from build123d import *

# Parameters (mm, degrees)
F0_R     = 14.25
F1_DEPTH = 83
F2_W     = 44.470418
F2_H     = 54.147916
F3_DEPTH = 12.5
F4_R     = 14.971262
F4_R_2   = 11
F5_DEPTH = 14


with BuildPart() as f1:
    # F0 (on Top) → F1 (new body)
    with BuildSketch(Plane.XY):
        with BuildLine():
            ThreePointArc((-11, 11.61895), (-6.324555, -14.696938), (16, 0))
            ThreePointArc((16, 0), (14.696938, 6.324555), (11, 11.61895))
            ThreePointArc((11, 11.61895), (0, 16), (-11, 11.61895))
        make_face()
        Circle(F0_R, mode=Mode.SUBTRACT)
        with BuildLine():
            ThreePointArc((-11, 76.61895), (0, 65.61895), (11, 76.61895))
            ThreePointArc((11, 76.61895), (10.797649, 78.719137), (10.198039, 80.742056))
            Line((10.198039, 80.742056), (8, 80.742056))
            ThreePointArc((8, 80.742056), (0, 67.61895), (-8, 80.742056))
            Line((-8, 80.742056), (-10.198039, 80.742056))
            ThreePointArc((-10.198039, 80.742056), (-10.797649, 78.719137), (-11, 76.61895))
        make_face()
        with BuildLine():
            ThreePointArc((-11, 11.61895), (0, 16), (11, 11.61895))
            Line((11, 11.61895), (11, 76.61895))
            ThreePointArc((11, 76.61895), (0, 65.61895), (-11, 76.61895))
            Line((-11, 76.61895), (-11, 11.61895))
        make_face()
    extrude(amount=F1_DEPTH)

    # F2 (on Right) → F3 (cut, symmetric)
    with BuildSketch(Plane.YZ):
        with Locations((33.410417, 41.327498)):
            Rectangle(F2_W, F2_H)
    extrude(amount=F3_DEPTH, both=True, mode=Mode.SUBTRACT)

    # F4 (on Top) → F5 (join)
    with BuildSketch(Plane.XY):
        Circle(F4_R)
        Circle(F4_R_2, mode=Mode.SUBTRACT)
    extrude(amount=F5_DEPTH)


solid = f1.part
Geometry check sheet. Reference: the model listing, model coordinates, mm. A direction names the side the tool comes from. Give positions to 0.01 mm unless a question says otherwise; leave off trailing zeros. Loops run counter-clockwise (first coordinate to the right, second up) from the corner with the lowest first, then second, coordinate; pieces in that order, holes last.
(1) Thickness scan on L1, parallel to Y at x = 0, z = 10.25; L2, parallel to Z at x = 4, y = 14; L3, parallel to X at y = 0, z = 28. Record the ranges inside material, lowest first.
From the geometry:
L1: y = -16 to -11, 11 to 67.62
L2: z = 0 to 14.25, 68.4 to 83
L3: x = -16 to -14.25, 14.25 to 16
(2) Depth check by flat-ended pin: pin 1 Ø1 at (y, z) = (12, 34.5) entering from -X; pin 2 Ø1.5 at (x, z) = (6, 41.5) entering from +Y; pin 3 Ø4 at (x, z) = (-11, 10.5) entering from -Y. Enter the tip coordinate at first touch or a pass-through.
From the geometry:
pin 1: passes through
pin 2: stops at y = 70.67
pin 3: stops at y = -13.23
(3) Section check A-A on y = 42. Record the cut outline in (x, z), then the cut area to 3 significant figures.
From the geometry:
outline: (-11, 0) - (11, 0) - (11, 14.25) - (-11, 14.25) - close; (-11, 68.4) - (11, 68.4) - (11, 83) - (-11, 83) - close
area: 635 mm2
(4) Release check for a two-part mould opening along Y. For faces 1 (the flat face through (0, 44, 83)), 2 (the cylindrical face through (0.258, 67.623, 40.919)), 3 (the cylindrical face through (-10.8, 78.7, 40.9)) record: released by +Y, released by -Y, zero draft, split by the parting line, or undercut.
From the geometry:
face 1: zero draft
face 2: undercut
face 3: released by +Y
(5) Set-up check for faces 4 (the flat face through (0, 33, 14.254)), 5 (the flat face through (-11, 59, 41)), 6 (the flat face through (11, 58, 41)): record each of +Z, -Z, +X, -X, +Y, -Y from which the full face is reachable in a straight line by a thin tool's end or side.
From the geometry:
face 4: +X, -X
face 5: +Z, -Z, -X, +Y
face 6: +Z, -Z, +X, +Y
(6) Section check D-D on x = 6. Record the cut outline in (y, z), then the cut area to 3 significant figures.
From the geometry:
outline: (-14.83, 0) - (-9.22, 0) - (-9.22, 14) - (-12.93, 14) - (-12.93, 83) - (-14.83, 83) - close; (9.22, 0) - (69.91, 0) - (69.91, 83) - (12.93, 83) - (12.93, 68.4) - (55.65, 68.4) - (55.65, 14.25) - (12.93, 14.25) - (12.93, 14) - (9.22, 14) - close
area: 2,680 mm2
(7) Section check C-C on x = 0. Record the cut outline in (y, z), then the cut area to 3 significant figures.
From the geometry:
outline: (-16, 0) - (-11, 0) - (-11, 14) - (-14.25, 14) - (-14.25, 83) - (-16, 83) - close; (11, 0) - (67.62, 0) - (67.62, 83) - (14.25, 83) - (14.25, 68.4) - (55.65, 68.4) - (55.65, 14.25) - (14.25, 14.25) - (14.25, 14) - (11, 14) - close
area: 2,420 mm2
(8) Section check B-B on z = 48. Record the cut outline in (x, y), then the cut area to 3 significant figures.
From the geometry:
outline: (-11.45, 11.18) arc R16 ccw (long way) to (16, 0) arc R16 ccw to (11.45, 11.18) - (8.84, 11.18) arc R14.25 cw (long way) to (-8.84, 11.18) - close; (-11, 55.65) - (11, 55.65) - (11, 76.62) arc R11 ccw to (10.2, 80.74) - (8, 80.74) arc R9 cw (long way) to (-8, 80.74) - (-10.2, 80.74) arc R11 ccw to (-11, 76.62) - close
area: 478 mm2
